```python
from build123d import *

# Parameters (mm, degrees)
SKETCH1_R           = 4
BOSS_EXTRUDE1_DEPTH = 40
SKETCH3_R           = 8
BOSS_EXTRUDE2_DEPTH = 20
SKETCH4_R           = 5
BOSS_EXTRUDE3_DEPTH = 108
SKETCH5_W           = 14
SKETCH5_H           = 2
BOSS_EXTRUDE4_DEPTH = 130
CUT_EXTRUDE1_REACH  = 26
SKETCH6_R           = 4


with BuildPart() as part:
    # Sketch1 → Boss-Extrude1 (new body, symmetric)
    with BuildSketch(Plane(origin=(0, 0, 0), x_dir=(1, 0, 0), z_dir=(0, 1, 0))):
        Circle(SKETCH1_R)
    extrude(amount=BOSS_EXTRUDE1_DEPTH, both=True)

    # Sketch3 → Boss-Extrude2 (add, symmetric)
    with BuildSketch(Plane(origin=(0, 0, 0), x_dir=(1, 0, 0), z_dir=(0, 1, 0))):
        Circle(SKETCH3_R)
    extrude(amount=BOSS_EXTRUDE2_DEPTH, both=True)

    # Sketch4 → Boss-Extrude3 (add)
    with BuildSketch(Plane(origin=(0, 0, 0), x_dir=(0, 0, -1), z_dir=(1, 0, 0))):
        Circle(SKETCH4_R)
    extrude(amount=BOSS_EXTRUDE3_DEPTH)

    # Sketch5 → Boss-Extrude4 (add)
    with BuildSketch(Plane(origin=(0, 0, 0), x_dir=(0.939692621, 0, 0.342020143), z_dir=(-0.342020143, 0, 0.939692621))):
        with Locations((0, -17)):
            Rectangle(SKETCH5_W, SKETCH5_H)
    extrude(amount=BOSS_EXTRUDE4_DEPTH)

    # Sketch6 → Cut-Extrude1 (cut, up to next)
    with BuildSketch(Plane(origin=(0, -16, 0), x_dir=(1, 0, 0), z_dir=(0, 1, 0)), mode=Mode.PRIVATE) as cut_extrude1_sk1:
        with Locations((-41.042417199, -112.763114494)):
            Circle(SKETCH6_R)
    cut_extrude1_tool1 = extrude(cut_extrude1_sk1.sketch, amount=-CUT_EXTRUDE1_REACH, mode=Mode.PRIVATE) & part.part
    add(cut_extrude1_tool1.solids().sort_by_distance((-41.042417, -16, 112.763114))[0], mode=Mode.SUBTRACT)


solid = part.part
```
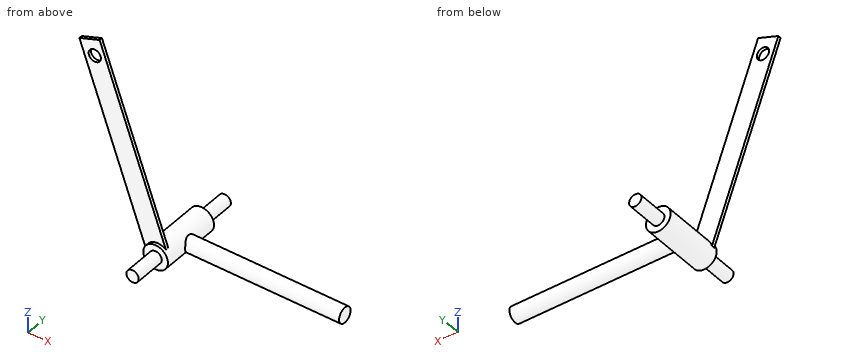
Geometry: final body of the model. Coordinates: model frame, mm. Give positions to 0.01 mm unless a question says otherwise; leave off trailing zeros. Write each loop counter-clockwise with the first axis right and the second up, starting at its lowest first coordinate (ties: lowest second). Pieces come first, ordered by that corner, then holes.
1. Section query B-B, the plane y = 11. Return loops of the section in (x, z).
2. Line query: probe 1 along X at (y, z) = (-17.5, 79); probe 2 along Z at (x, y) = (11.5, -3); probe 3 along Z at (x, y) = (-2, -6). Output: solid intervals per line, ascending.
3. Section query A-A, the plane x = 0. Return loops of the section in (y, z).
4. Section query D-D, the plane z = 13. Return loops of the section in (x, y), then the cut area to 3 significant figures.
5. Pin query (flat end, axial travel): P1, Ø17.5, axis at x = -3.5, z = -3, coming from the +Y side; P2, Ø5, axis at y = -14.5, z = 43.5, coming from the -X side; P3, Ø5, axis at x = -41.04, z = 112.76, coming from the +Y side; P4, Ø17, axis at x = -34, z = 89.5, coming from the +Y side. Return the tip coordinate at first contact, or that it passes through.
6. Section query C-C, the plane x = 87.5. Return loops of the section in (y, z).
Computed:
1. outline: circle Ø16 at (0, 0)
2. probe 1: x = -36.2 to -21.3
2. probe 2: z = -4 to 4
2. probe 3: z = -7.75 to 7.75
3. outline: (-40, -4) - (-20, -4) - (-20, -8) - (20, -8) - (20, -4) - (40, -4) - (40, 4) - (20, 4) - (20, 8) - (-16, 8) - (-16, 20.47) - (-18, 20.47) - (-18, 8) - (-20, 8) - (-20, 4) - (-40, 4) - close
4. outline: (-12.18, -18) - (2.72, -18) - (2.72, -16) - (-12.18, -16) - close
4. area: 29.8 mm2
5. P1: stops at y = 40
5. P2: stops at x = -24.01
5. P3: passes through
5. P4: stops at y = -16
6. outline: circle Ø10 at (0, 0)
